Job drawing, mm, ordinate dimensions from the low corner. One solid piece. Give positions to 0.01 mm unless a question says otherwise; leave off trailing zeros. Loops run counter-clockwise (first coordinate to the right, second up) from the corner with the lowest first, then second, coordinate; pieces in that order, holes last. Notation, with made-up numbers: (55.25, 49) -> (92.25, 49) arc R20 ccw to (92.25, 57) -> close; hole circle Ø10 at (53, 42). An arc over 180 degrees is marked (long way). Use one line per item in the form item = value.
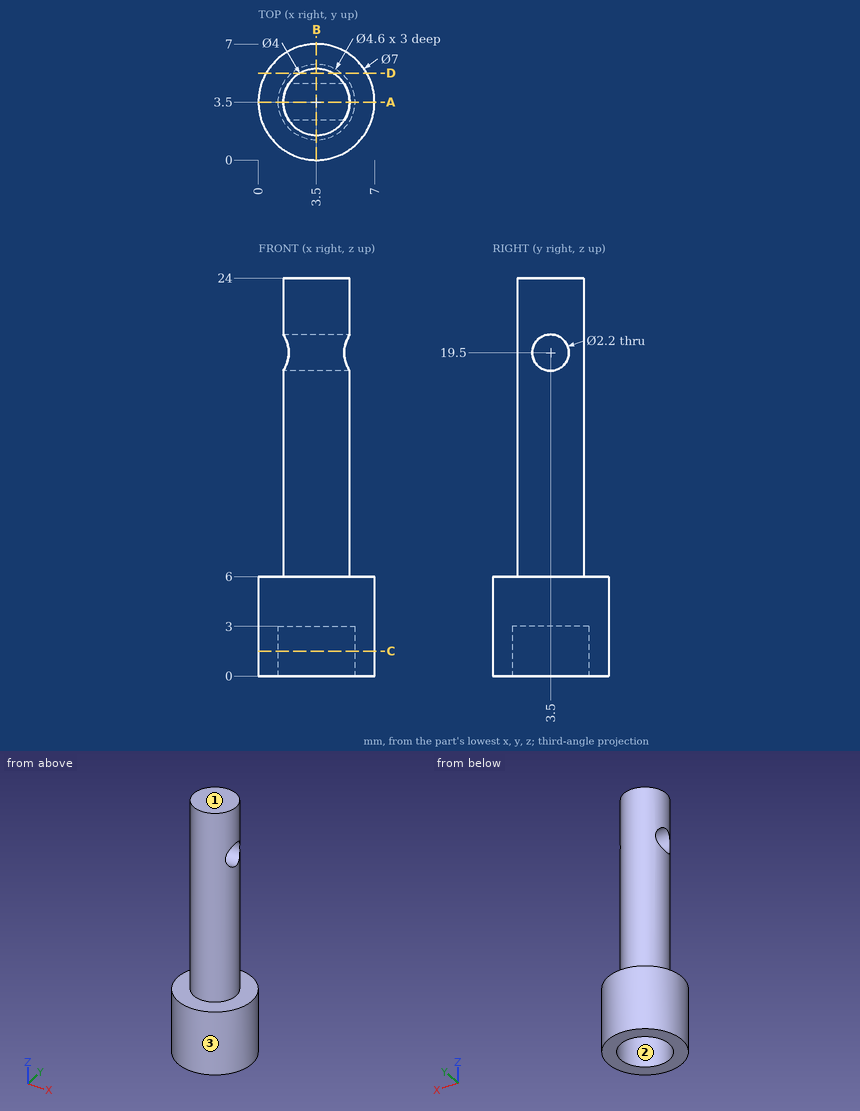
1. Drop flat-ended pins along their axis: P1, Ø1, axis at x = 4.5, z = 2.5, coming from the +Y side; P2, Ø2, axis at x = 6, z = 9.5, coming from the +Y side; P3, Ø1, axis at x = 6, z = 5.5, coming from the +Y side. Give the stop position or say it passes through.
Result sheet:
P1 = 6.96
P2 = 4.82
P3 = 6.37
2. Cut at D-D, the plane y = 5.25. Write the cut outline in (x, z), then the cut area to 3 significant figures.
Result sheet:
outline = (0.47, 0) -> (2.01, 0) -> (2.01, 3) -> (4.99, 3) -> (4.99, 0) -> (6.53, 0) -> (6.53, 6) -> (4.47, 6) -> (4.47, 24) -> (2.53, 24) -> (2.53, 6) -> (0.47, 6) -> close
area = 62.3 mm^2
3. Drill centre lines: line 1 (Y direction, x = 3.5, z = 1.7); line 2 (Z direction, x = 3.15, y = 3.5); line 3 (Z direction, x = 5.75, y = 1). Where is each one in solid material? Low to high.
Result sheet:
line_1 = 0 to 1.2, 5.8 to 7
line_2 = 3 to 18.4, 20.6 to 24
line_3 = 0 to 6
4. Cut at B-B, the plane x = 3.5. Write the cut outline in (y, z).
Result sheet:
outline = (0, 0) -> (1.2, 0) -> (1.2, 3) -> (5.8, 3) -> (5.8, 0) -> (7, 0) -> (7, 6) -> (5.5, 6) -> (5.5, 24) -> (1.5, 24) -> (1.5, 6) -> (0, 6) -> close; hole circle Ø2.2 at (3.5, 19.5)
5. Cut at C-C, the plane z = 1.5. Write the cut outline in (x, y), then the cut area to 3 significant figures.
Result sheet:
outline = circle Ø7 at (3.5, 3.5); hole circle Ø4.6 at (3.5, 3.5)
area = 21.9 mm^2
6. Cut at A-A, the plane y = 3.5. Write the cut outline in (x, z), then the cut area to 3 significant figures.
Result sheet:
outline = (0, 0) -> (1.2, 0) -> (1.2, 3) -> (5.8, 3) -> (5.8, 0) -> (7, 0) -> (7, 6) -> (5.5, 6) -> (5.5, 18.4) -> (1.5, 18.4) -> (1.5, 6) -> (0, 6) -> close; (1.5, 20.6) -> (5.5, 20.6) -> (5.5, 24) -> (1.5, 24) -> close
area = 91.4 mm^2
7. Mould opens along Y. For the marked faces 1, 2 and 3 say: pulls with the +Y half, pulls with the -Y half, needs draft (parallel to the pull), parting line crosses it, or undercut.
Result sheet:
face_1 = needs draft
face_2 = undercut
face_3 = parting line crosses it
